Geometry check sheet. Reference: drawing and pictorial views, mm from the part's lowest x, y, z. A direction names the side the tool comes from. Coordinates: 2 decimals unless noted, no trailing zeros. Write each loop counter-clockwise with the first axis right and the second up, starting at its lowest first coordinate (ties: lowest second). Pieces come first, ordered by that corner, then holes. Notation, with made-up numbers: (76, 41.5) -> (85, 41.5) arc R35 cw to (85, 80.5) -> close; hole circle Ø7 at (12, 63.5). An arc over 180 degrees is marked (long way). Use a Markdown table: item, result. Add a question column.
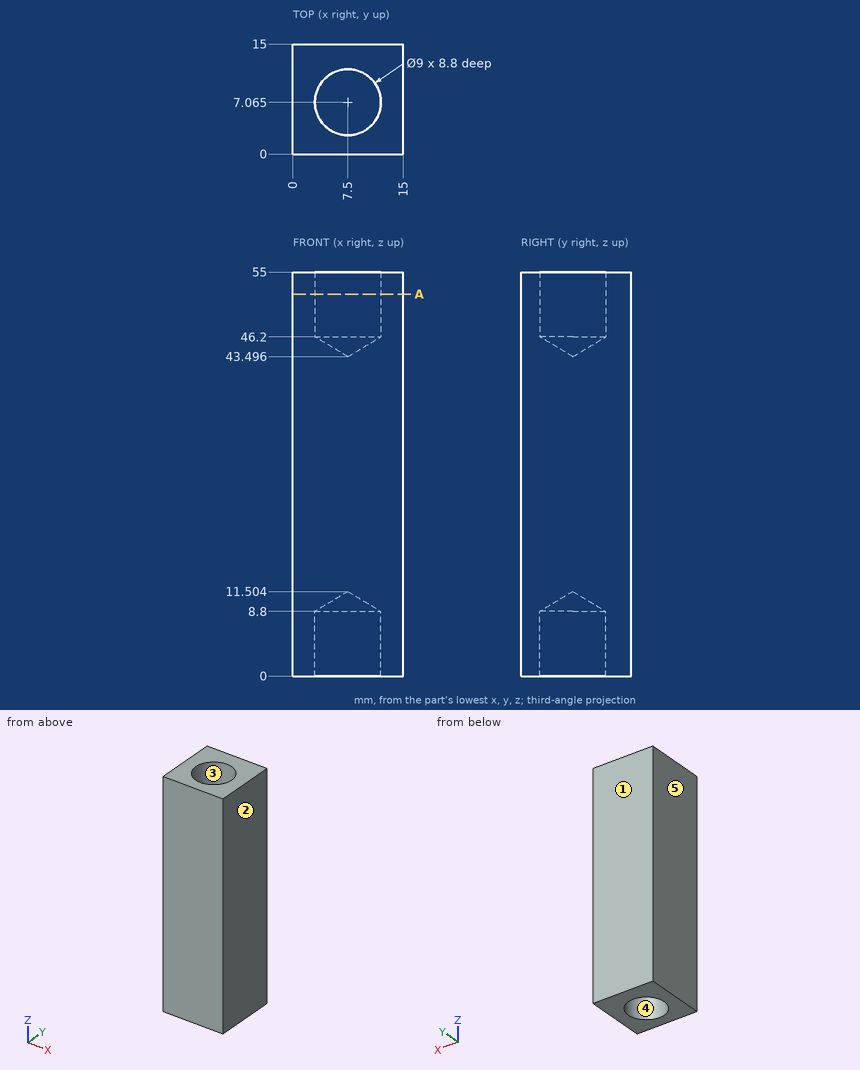
1) Set-up check for the marked faces 4 and 5: record each of +Z, -Z, +X, -X, +Y, -Y from which the full face is reachable in a straight line by a thin tool's end or side.
2) Thickness scan on L1, parallel to Y at x = 7.5, z = 51.5 (1 decimal); L2, parallel to X at y = 3.5, z = 7 (1 decimal); L3, parallel to Y at x = 9, z = 47. Record the ranges inside material, lowest first.
3) Gauge pin test, flat ends, axial feed: pin 1 (2 mm diameter, centred on x = 7.5, y = 10, fed in from -Z); pin 2 (5.5 mm diameter, centred on x = 7.5, y = 7.06, fed in from +Z). Record the tip position at first contact, or that the pin passes through.
4) Cross-section at A-A on z = 52. Record the boundary of the cut face in (x, y) (1 decimal).
5) Release check for a two-part mould opening along Y. For the marked faces 1, 2 and 3 record: released by +Y, released by -Y, zero draft, split by the parting line, or undercut.
Returned:
| question | item | result |
|---|---|---|
| 1 | face 4 | -Z |
| 1 | face 5 | +Z, -Z, -X, +Y, -Y |
| 2 | L1 | y = 0 to 2.6, 11.6 to 15 |
| 2 | L2 | x = 0 to 4.8, 10.2 to 15 |
| 2 | L3 | y = 0 to 2.82, 11.31 to 15 |
| 3 | pin 1 | stops at z = 9.14 |
| 3 | pin 2 | stops at z = 45.15 |
| 4 | outline | (0, 0) -> (15, 0) -> (15, 15) -> (0, 15) -> close; hole circle Ø9 at (7.5, 7.1) |
| 5 | face 1 | released by +Y |
| 5 | face 2 | zero draft |
| 5 | face 3 | undercut |
